from build123d import *

# Parameters (mm, degrees)
SKETCH1_R           = 2.5
SKETCH1_R_2         = 1.5
BOSS_EXTRUDE1_DEPTH = 4
SKETCH2_R           = 17.5
SKETCH2_R_2         = 15
BOSS_EXTRUDE2_DEPTH = 4
BOSS_EXTRUDE5_DEPTH = 1
FILLET1_R           = 2
FILLET2_R           = 2
SKETCH4_R           = 22.5
SKETCH4_R_2         = 17.5
BOSS_EXTRUDE6_DEPTH = 4.5
FILLET3_R           = 4


with BuildPart() as part:
    # Sketch1 → Boss-Extrude1 (new, symmetric)
    with BuildSketch(Plane.XY):
        Circle(SKETCH1_R)
        Circle(SKETCH1_R_2, mode=Mode.SUBTRACT)
    extrude(amount=BOSS_EXTRUDE1_DEPTH, both=True)



with BuildPart() as body_2:
    # Sketch2 → Boss-Extrude2 (new, symmetric)
    with BuildSketch(Plane.XY):
        Circle(SKETCH2_R)
        Circle(SKETCH2_R_2, mode=Mode.SUBTRACT)
    extrude(amount=BOSS_EXTRUDE2_DEPTH, both=True)


with BuildPart() as part_1:
    add(part.part)

    add(body_2.part)  # Boss-Extrude5 merges body 2
    # Sketch3 → Boss-Extrude5 (add, symmetric)
    with BuildSketch(Plane.XY):
        with BuildLine():
            Line((-1, 2.291287847), (-1, 14.966629547))
            ThreePointArc((-1, 14.966629547), (0, 15), (1, 14.966629547))
            Line((1, 14.966629547), (1, 2.291287847))
            ThreePointArc((1, 2.291287847), (0, 2.5), (-1, 2.291287847))
        make_face()
        with BuildLine():
            Line((1.484313483, 2.011669328), (12.461481397, 8.349340177))
            ThreePointArc((12.461481397, 8.349340177), (12.990381057, 7.5), (13.461481397, 6.61728937))
            Line((13.461481397, 6.61728937), (2.484313483, 0.27961852))
            ThreePointArc((2.484313483, 0.27961852), (2.165063509, 1.25), (1.484313483, 2.011669328))
        make_face()
        with BuildLine():
            Line((2.484313483, -0.27961852), (13.461481397, -6.61728937))
            ThreePointArc((13.461481397, -6.61728937), (12.990381057, -7.5), (12.461481397, -8.349340177))
            Line((12.461481397, -8.349340177), (1.484313483, -2.011669328))
            ThreePointArc((1.484313483, -2.011669328), (2.165063509, -1.25), (2.484313483, -0.27961852))
        make_face()
        with BuildLine():
            Line((1, -2.291287847), (1, -14.966629547))
            ThreePointArc((1, -14.966629547), (0, -15), (-1, -14.966629547))
            Line((-1, -14.966629547), (-1, -2.291287847))
            ThreePointArc((-1, -2.291287847), (0, -2.5), (1, -2.291287847))
        make_face()
        with BuildLine():
            Line((-1.484313483, -2.011669328), (-12.461481397, -8.349340177))
            ThreePointArc((-12.461481397, -8.349340177), (-12.990381057, -7.5), (-13.461481397, -6.61728937))
            Line((-13.461481397, -6.61728937), (-2.484313483, -0.27961852))
            ThreePointArc((-2.484313483, -0.27961852), (-2.165063509, -1.25), (-1.484313483, -2.011669328))
        make_face()
        with BuildLine():
            Line((-2.484313483, 0.27961852), (-13.461481397, 6.61728937))
            ThreePointArc((-13.461481397, 6.61728937), (-12.990381057, 7.5), (-12.461481397, 8.349340177))
            Line((-12.461481397, 8.349340177), (-1.484313483, 2.011669328))
            ThreePointArc((-1.484313483, 2.011669328), (-2.165063509, 1.25), (-2.484313483, 0.27961852))
        make_face()
    extrude(amount=BOSS_EXTRUDE5_DEPTH, both=True)

    # Fillet1
    fillet1_edges = [part_1.edges().sort_by_distance(p)[0] for p in [
        (-15, 0, -4),
        (-15, 0, 4),
    ]]
    fillet(fillet1_edges, radius=FILLET1_R)

    # Fillet2
    fillet2_edges = [part_1.edges().sort_by_distance(p)[0] for p in [
        (-1, -8.628958697, 1),
        (6.97289744, -5.180504752, 1),
        (7.97289744, 3.448453945, 1),
        (1, 8.628958697, 1),
        (-6.97289744, 5.180504752, 1),
        (-7.97289744, -3.448453945, 1),
    ]]
    fillet(fillet2_edges, radius=FILLET2_R - 0.0001)  # a hair under: the kernel refuses the full size

    # Sketch4 → Boss-Extrude6 (add, symmetric)
    with BuildSketch(Plane.XY):
        Circle(SKETCH4_R)
        Circle(SKETCH4_R_2, mode=Mode.SUBTRACT)
    extrude(amount=BOSS_EXTRUDE6_DEPTH, both=True)

    # Fillet3
    fillet3_edges = [part_1.edges().sort_by_distance(p)[0] for p in [
        (-22.5, 0, 4.5),
        (-22.5, 0, -4.5),
    ]]
    fillet(fillet3_edges, radius=FILLET3_R)


solid = part_1.part
Read the model definition and answer for the solid it produces. Units are mm, in the model's axes. A direction names the side the tool comes from. Give positions to 0.01 mm unless a question says otherwise; leave off trailing zeros. Write each loop counter-clockwise with the first axis right and the second up, starting at its lowest first coordinate (ties: lowest second). Pieces come first, ordered by that corner, then holes. Notation, with made-up numbers: (3, -24.5) - (39, -24.5) arc R21 cw to (39, -16.5) - close; hole circle Ø2 at (64, -19.75). An arc over 180 degrees is marked (long way). Answer in a Markdown table with one row per item. Add a question column.
Item 1: Section C-C, the plane z = -3 is taken. Write down the section's boundary in (x, y) (1 decimal), and give its area (3 significant figures).
Item 2: Flat-ended cylindrical pins translate along their axes: P1, Ø1.9, axis at x = -5.5, y = 4.5, coming from the +Z side; P2, Ø0.6, axis at y = -9.5, z = 0, coming from the +X side; P3, Ø4, axis at x = -1, y = 1, coming from the +Z side. Find the tip coordinate at first contact, or state that the pin passes through.
Item 3: A tool of negligible diameter and unlimited length cuts with its end or side. For faces 4 (the face through (0.43, 8.56, 0.4)), 5 (the face through (-13.887, -10.648, -4.254)), 6 (the face through (7.896, -3.404, -0.014)), from which of +Z, -Z, +X, -X, +Y, -Y can it reach the whole face along a straight path? Write none if from no direction.
Item 4: Determine the mould class of faces 1 (the face through (10.382, -19.961, 0.007)), 2 (the face through (0, -9, -1)), 3 (the face through (-11, -14, 4.5)) for opening direction X: pulls with the +X half, pulls with the -X half, needs draft (parallel to the pull), parting line crosses it, or undercut.
Item 5: Section A-A, the plane y = -4.5 is taken. Count the separate pieces of the cut face and the enclosed holes in it, and give its area (3 significant figures).
Item 6: Find the intervals of material crossed by L1, parallel to Y at x = 0, z = -0.75; L2, parallel to X at y = -9, z = 0; L3, parallel to Y at x = 2, z = 1.5, in increasing order.
Recorded:
| question | item | result |
|---|---|---|
| 1 | outline | circle Ø43.2 at (0, 0); circle Ø5 at (0, 0); hole circle Ø30.5 at (0, 0); hole circle Ø3 at (0, 0) |
| 1 | area | 749 mm2 |
| 2 | P1 | stops at z = 0.6 |
| 2 | P2 | stops at x = 20.53 |
| 2 | P3 | stops at z = 4 |
| 3 | face 4 | +Z |
| 3 | face 5 | -Z |
| 3 | face 6 | +Z, -Z |
| 4 | face 1 | parting line crosses it |
| 4 | face 2 | undercut |
| 4 | face 3 | needs draft |
| 5 | separate pieces | 5 |
| 5 | enclosed holes | 0 |
| 5 | area | 132 mm2 |
| 6 | L1 | y = -22.49 to -1.5, 1.5 to 22.49 |
| 6 | L2 | x = -20.62 to -12, -0.73 to 1, 12 to 20.62 |
| 6 | L3 | y = -22.28 to -14.87, -1.5 to 1.5, 14.87 to 22.28 |
